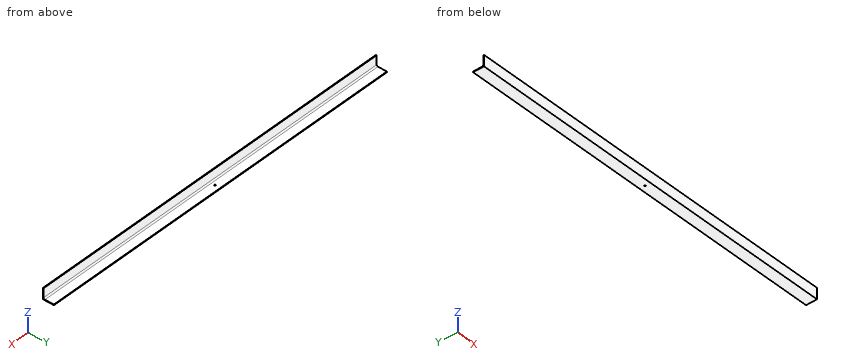
```python
from build123d import *

# Parameters (mm, degrees)
BASE_DEPTH          = 1215
SKETCH_1_R          = 4
CUT_EXTRUDE_1_DEPTH = 5


with BuildPart() as part:
    # Sketch1 → Base (new body, symmetric)
    with BuildSketch(Plane.YZ):
        with BuildLine():
            Line((0, 70), (0, 0))
            Line((0, 0), (70, 0))
            Line((70, 0), (70, 2.666666667))
            ThreePointArc((70, 2.666666667), (69.609475708, 3.609475708), (68.666666667, 4))
            Line((68.666666667, 4), (12, 4))
            ThreePointArc((12, 4), (6.343145751, 6.343145751), (4, 12))
            Line((4, 12), (4, 68.666666667))
            ThreePointArc((4, 68.666666667), (3.609475708, 69.609475708), (2.666666667, 70))
            Line((2.666666667, 70), (0, 70))
        make_face()
    extrude(amount=BASE_DEPTH, both=True)

    # 草图1 → 切除-拉伸1 (cut, through all)
    with BuildSketch(Plane.XY.offset(4)):
        with Locations((0, 35)):
            Circle(SKETCH_1_R)
    extrude(amount=-CUT_EXTRUDE_1_DEPTH, mode=Mode.SUBTRACT)


solid = part.part
```
Input: part model. Units: mm. Frame: model coordinates. Coordinates: 2 decimals unless noted, no trailing zeros. Loops run counter-clockwise (first coordinate to the right, second up) from the corner with the lowest first, then second, coordinate; pieces in that order, holes last. Notation, with made-up numbers: (32, 57.25) -> (39, 57.25) arc R13 ccw to (39, 71.25) -> close; hole circle Ø2 at (68, 62). An arc over 180 degrees is marked (long way). Use a Markdown table: item, result.
1) Material intervals for line 1 along Y through (x, z) = (0, 2); line 2 along Y through (x, z) = (-331.5, 49), sorted ascending. Write a range as from..to.
Results found:
| item | result |
|---|---|
| line 1 | y = 0..31, 39..70 |
| line 2 | y = 0..4 |
2) Cut plane A-A (x = 784). Return the cut outline in (y, z), then the cut area to 3 significant figures.
Results found:
| item | result |
|---|---|
| outline | (0, 0) -> (70, 0) -> (70, 2.67) arc R1.33 ccw to (68.67, 4) -> (12, 4) arc R8 cw to (4, 12) -> (4, 68.67) arc R1.33 ccw to (2.67, 70) -> (0, 70) -> close |
| area | 557 mm2 |
3) Contact query for flat-ended pins moving along their axis: pin 1 (12 mm diameter, centred on y = 12, z = 19.5, fed in from +X); pin 2 (17 mm diameter, centred on x = 498, z = 46, fed in from +Y); pin 3 (10.5 mm diameter, centred on x = 0, y = 35, fed in from +Z). Output: stop coordinate, or through.
Results found:
| item | result |
|---|---|
| pin 1 | passes through |
| pin 2 | stops at y = 4 |
| pin 3 | stops at z = 4 |
4) Cut plane B-B (z = 41). Return the cut outline in (x, y), then the cut area to 3 significant figures.
Results found:
| item | result |
|---|---|
| outline | (-1215, 0) -> (1215, 0) -> (1215, 4) -> (-1215, 4) -> close |
| area | 9,720 mm2 |
